Design review of the part built by this model. Coordinates are the model's own, in mm. Face numbers are marked on the shaded views. A direction names the side the tool comes from. Coordinates: 2 decimals unless noted, no trailing zeros. Loops run counter-clockwise (first coordinate to the right, second up) from the corner with the lowest first, then second, coordinate; pieces in that order, holes last.
Q1. Machinability: for the marked faces 1 and 2, which of the approach directions +Z, -Z, +X, -X, +Y, -Y give a long, thin tool a straight path to every point of the face, cutting with its end or side? Answer none if there is none.
Q2. Add section B-B on z = 49.5. Give the boundary of the cut face in (x, y), and give its area (3 significant figures).
Q3. Add section A-A on x = 72. Give the boundary of the cut face in (y, z), and give its area (3 significant figures).
Q4. Wall thickness on probe 1 along Z at (x, y) = (90, 16); probe 2 along Y at (x, z) = (62.5, 49); probe 3 along X at (y, z) = (34, 26): over which ranges is each line inside the solid? List them lowest first.
Q5. For P1, Ø12.5, axis at x = 89, z = 32.5, coming from the +Y side; P2, Ø5, axis at y = 17.5, z = 15.5, coming from the -X side; P3, Ø7.5, axis at x = 63.5, z = 18, coming from the +Y side; P4, Ø3, axis at y = 6.5, z = 45, coming from the +X side, all flat-tipped, find the tip position at first contact; note any pin that passes through.
Q6. Add section D-D on y = 6. Give the boundary of the cut face in (x, z), and give its area (3 significant figures).
Q7. Add section C-C on y = 18. Give the boundary of the cut face in (x, z), and give its area (4 significant figures).
```python
from build123d import *

# Parameters (mm, degrees)
BOSS_EXTRUDE1_DEPTH = 100
SKETCH1_3_W         = 55
SKETCH1_3_H         = 40
BOSS_EXTRUDE2_DEPTH = 75
CUT_EXTRUDE1_DEPTH  = 75


with BuildPart() as part:
    # Sketch1 → Boss-Extrude1 (new body)
    with BuildSketch(Plane(origin=(0, 0, 0), x_dir=(0, 0, -1), z_dir=(1, 0, 0))):
        Polygon((20, 40), (0, 40), (0, 0), (-55, 0), (-55, -15), (20, -15), align=None)
    extrude(amount=BOSS_EXTRUDE1_DEPTH)

    # Sketch1<3> → Boss-Extrude2 (add)
    with BuildSketch(Plane(origin=(0, 0, 0), x_dir=(0, 0, -1), z_dir=(1, 0, 0))):
        with Locations((-27.5, 20)):
            Rectangle(SKETCH1_3_W, SKETCH1_3_H)
    extrude(amount=BOSS_EXTRUDE2_DEPTH)

    # Sketch4 → Cut-Extrude1 (cut, along a direction that is not the sketch's normal)
    with BuildSketch(Plane(origin=(42.394160584, 31.795620438, 19.270072993), x_dir=(-0.27339445046936345, -0.20504583785202254, 0.9397934234884372), z_dir=(-0.7518347387907499, -0.5638760540930621, -0.34174306308670427))):
        Polygon((38.018915768, 20), (-20.504583785, 5), (-20.504583785, -45), (38.018915768, -30), align=None)
    extrude(amount=-CUT_EXTRUDE1_DEPTH, dir=(-1, 0, 0), mode=Mode.SUBTRACT)


solid = part.part
```
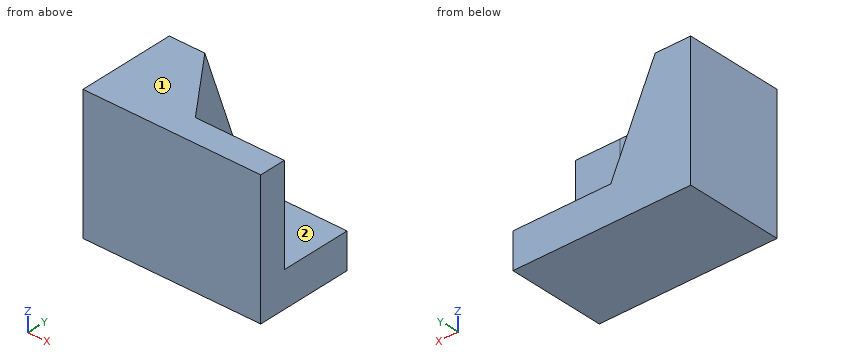
Entries:
1. face 1: +Z, +X, -X, +Y, -Y
1. face 2: +Z, +X, +Y
2. outline: (0, -15) - (100, -15) - (100, 0) - (52.5, 0) - (22.5, 40) - (0, 40) - close
2. area: 3,000 mm2
3. outline: (-15, -20) - (40, -20) - (40, 0) - (4, 0) - (0, 6.6) - (0, 55) - (-15, 55) - close
3. area: 1,940 mm2
4. probe 1: z = -20 to 0
4. probe 2: y = -15 to 0
4. probe 3: x = 0 to 37.68
5. P1: stops at y = 0
5. P2: stops at x = 0
5. P3: stops at y = 9.92
5. P4: stops at x = 50.99
6. outline: (0, -20) - (100, -20) - (100, 0) - (70.5, 0) - (45.5, 55) - (0, 55) - close
6. area: 5,190 mm2
7. outline: (0, -20) - (100, -20) - (100, 0) - (61.5, 0) - (36.5, 55) - (0, 55) - close
7. area: 4,695 mm2
